Design review of the part built by this model. Coordinates are the model's own, in mm. A direction names the side the tool comes from. Round coordinates to 2 decimals unless told otherwise and drop trailing zeros. Write each loop counter-clockwise with the first axis right and the second up, starting at its lowest first coordinate (ties: lowest second). Pieces come first, ordered by that corner, then holes. Notation, with made-up numbers: (-36, 3.25) -> (-26, 3.25) arc R9 cw to (-26, 16.25) -> close; hole circle Ø9 at (-17.5, -4.5). An arc over 180 degrees is marked (long way). One line per question, with ' | ' between items. Start each with the question number.
1) Consider section C-C (x = 0). Give the boundary of the cut face in (y, z), then the cut area to 3 significant figures.
2) For probe 1 along Z at (x, y) = (5.5, 0.3); probe 2 along X at (y, z) = (1.3, -2.25), list the stretches that pass through material, from the lowest coordinate up.
3) Consider section B-B (z = -6.7). Give the boundary of the cut face in (x, y), then the cut area to 3 significant figures.
4) Consider section D-D (z = 4). Give the boundary of the cut face in (x, y).
5) Consider section A-A (y = 0.9). Give the boundary of the cut face in (x, z).
6) For faces 1 (the flat face through (0, 1, 6)), 2 (the flat face through (-0.04, 0, -6.15)), list the 3-axis set-ups (+Z, -Z, +X, -X, +Y, -Y) from which the entire face can be reached by the end or side of a thin tool; tool diameter is ignored.
7) Mouldability with a two-part tool opening along X and no side actions: class faces 3 (the flat face through (-7.5, 1, 0)), 4 (the cylindrical face through (-0.54, 0.74, -2.44)), 5 (the flat face through (7.5, 1, 0)) as +X half, -X half, draft (parallel to the pull), parting line (faces both ways), or undercut.
```python
from build123d import *

# Parameters (mm, degrees)
SKETCH1_W           = 15
SKETCH1_H           = 15
BOSS_EXTRUDE1_DEPTH = 3
SKETCH2_W           = 12
SKETCH2_H           = 12
SKETCH2_R           = 2.5
CUT_EXTRUDE1_DEPTH  = 1.5
SKETCH3_R           = 0.75
CUT_EXTRUDE2_DEPTH  = 2


with BuildPart() as part:
    # Sketch1 → Boss-Extrude1 (new body)
    with BuildSketch(Plane(origin=(0, 0, 0), x_dir=(1, 0, 0), z_dir=(0, 1, 0))):
        Rectangle(SKETCH1_W, SKETCH1_H)
    extrude(amount=BOSS_EXTRUDE1_DEPTH)

    # Sketch2 → Cut-Extrude1 (cut)
    with BuildSketch(Plane.XZ):
        Rectangle(SKETCH2_W, SKETCH2_H)
        Circle(SKETCH2_R, mode=Mode.SUBTRACT)
    extrude(amount=-CUT_EXTRUDE1_DEPTH, mode=Mode.SUBTRACT)

    # Sketch3 → Cut-Extrude2 (cut)
    with BuildSketch(Plane.XZ):
        with Locations((-6.7, 6.7)):
            Circle(SKETCH3_R)
        with Locations((6.7, 6.7)):
            Circle(SKETCH3_R)
        with Locations((6.7, -6.7)):
            Circle(SKETCH3_R)
        with Locations((-6.7, -6.7)):
            Circle(SKETCH3_R)
    extrude(amount=-CUT_EXTRUDE2_DEPTH, mode=Mode.SUBTRACT)


solid = part.part
```
From the geometry:
1) outline: (0, -7.5) -> (3, -7.5) -> (3, 7.5) -> (0, 7.5) -> (0, 6) -> (1.5, 6) -> (1.5, 2.5) -> (0, 2.5) -> (0, -2.5) -> (1.5, -2.5) -> (1.5, -6) -> (0, -6) -> close | area: 34.5 mm2
2) probe 1: z = -7.5 to -6, 6 to 7.5 | probe 2: x = -7.5 to -6, -1.09 to 1.09, 6 to 7.5
3) outline: (-7.5, 0) -> (-7.45, 0) -> (-7.45, 2) -> (-5.95, 2) -> (-5.95, 0) -> (5.95, 0) -> (5.95, 2) -> (7.45, 2) -> (7.45, 0) -> (7.5, 0) -> (7.5, 3) -> (-7.5, 3) -> close | area: 39.0 mm2
4) outline: (-7.5, 0) -> (-6, 0) -> (-6, 1.5) -> (6, 1.5) -> (6, 0) -> (7.5, 0) -> (7.5, 3) -> (-7.5, 3) -> close
5) outline: (-7.5, -7.5) -> (7.5, -7.5) -> (7.5, 7.5) -> (-7.5, 7.5) -> close; circle Ø5 at (0, 0); hole circle Ø1.5 at (-6.7, -6.7); hole circle Ø1.5 at (-6.7, 6.7); hole (-6, -6) -> (6, -6) -> (6, 6) -> (-6, 6) -> close; hole circle Ø1.5 at (6.7, -6.7); hole circle Ø1.5 at (6.7, 6.7)
6) face 1: -Y | face 2: +Z, -Z, +X, -X, -Y
7) face 3: -X half | face 4: undercut | face 5: +X half
